Input: part model. Units: mm. Frame: model coordinates. Face numbers are marked on the shaded views. Give positions to 0.01 mm unless a question says otherwise; leave off trailing zeros. Loops run counter-clockwise (first coordinate to the right, second up) from the corner with the lowest first, then second, coordinate; pieces in that order, holes last. Notation, with made-up numbers: M -13,38.5 L 24,38.5 A34 cw 24,77.5 Z; hole C -37.5,45.5 d2. An arc over 180 degrees is marked long. One line per item, written item: value. Start each with the question number.
(1) Pull-direction query (X, two-part tool) for the marked faces 1, 2 and 3; classes: released by +X, released by -X, zero draft, split by the parting line, or undercut.
(2) Pin query (flat end, axial travel): P1, Ø5, axis at x = -11, z = 2, coming from the -Y side; P2, Ø1, axis at x = 9.5, z = 1.5, coming from the -Y side; P3, Ø5, axis at x = -2, z = 0.5, coming from the -Y side; P4, Ø10, axis at x = 5.5, y = -0.5, coming from the -Z side. Return the tip coordinate at first contact, or that it passes through.
(3) Ray query, line 1 along Y through (x, z) = (0, -2.75); line 2 along X through (y, z) = (2, 4.25); line 3 along X through (y, z) = (1.5, -3.75). Return the intervals inside material, ascending. Write a range as from..to.
(4) Section C-C on z = 2. Output: boundary loops of the cut face in (x, y), plus the area to 3 significant figures.
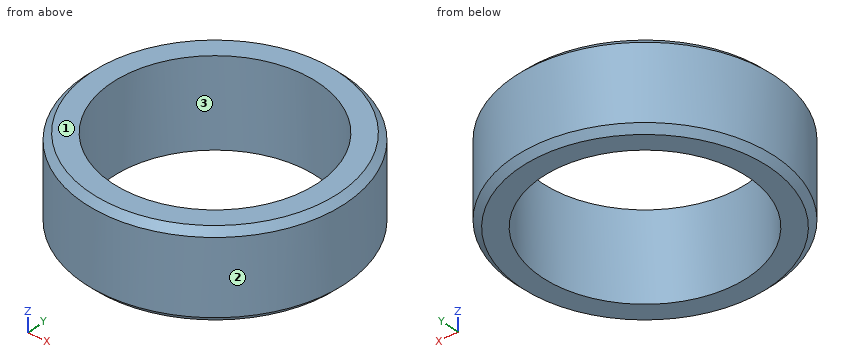
```python
from build123d import *

# Parameters (mm, degrees)
BOSS_EXTRUDE1_DEPTH      = 7.9375
BOSS_EXTRUDE1_DEPTH_BACK = 7.9375
SKETCH3_R                = 19.05
SKETCH3_R_2              = 9.525
CHAMFER1_SIZE            = 0.9525
SKETCH4_R                = 19.05
CUT_EXTRUDE1_DEPTH       = 3.175
SKETCH5_R                = 15.0495
CUT_EXTRUDE2_DEPTH       = 30.784140075
CHAMFER2_SIZE            = 0.9525


with BuildPart() as part:
    # Sketch3 → Boss-Extrude1 (new, two sides: drawn at the far end of the back side and taken through both)
    with BuildSketch(Plane.XY.offset(-BOSS_EXTRUDE1_DEPTH_BACK)):
        Circle(SKETCH3_R)
        Circle(SKETCH3_R_2, mode=Mode.SUBTRACT)
    extrude(amount=BOSS_EXTRUDE1_DEPTH + BOSS_EXTRUDE1_DEPTH_BACK)

    # Chamfer1
    chamfer1_edges = [part.edges().sort_by_distance(p)[0] for p in [
        (-19.05, 0, -7.9375),
        (-9.525, 0, -7.9375),
        (-19.05, 0, 7.9375),
        (-9.525, 0, 7.9375),
    ]]
    chamfer(chamfer1_edges, length=CHAMFER1_SIZE)

    # Sketch4 → Cut-Extrude1 (cut)
    with BuildSketch(Plane.XY.offset(7.9375)):
        Circle(SKETCH4_R)
    extrude(amount=-CUT_EXTRUDE1_DEPTH, mode=Mode.SUBTRACT)

    # Sketch5 → Cut-Extrude2 (cut, through all)
    with BuildSketch(Plane.XY.offset(4.7625)):
        Circle(SKETCH5_R)
    extrude(amount=-CUT_EXTRUDE2_DEPTH, mode=Mode.SUBTRACT)

    # Chamfer2
    chamfer2_edges = [part.edges().sort_by_distance(p)[0] for p in [
        (-19.05, 0, 4.7625),
    ]]
    chamfer(chamfer2_edges, length=CHAMFER2_SIZE)


solid = part.part
```
Output values:
1. face 1: zero draft
1. face 2: split by the parting line
1. face 3: undercut
2. P1: stops at y = -17.05
2. P2: stops at y = -16.79
2. P3: stops at y = -19.05
2. P4: passes through
3. line 1: y = -19.05..-15.05, 15.05..19.05
3. line 2: x = -18.5..-14.92, 14.92..18.5
3. line 3: x = -18.99..-14.97, 14.97..18.99
4. outline: C 0,0 d38.1; hole C 0,0 d30.1
4. area: 429 mm²
